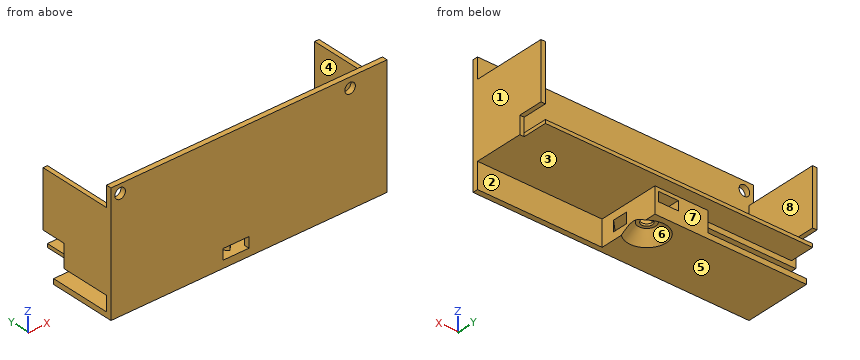
Autodesk Inventor part; units mm, degrees
ref_plane "Work Plane1" through (-11.25, -9.75, 3.625) normal (0, 0, -1) x (-1, 0, 0)
ref_plane "YZ Plane" through (0, 0, 0) normal (1, 0, 0) x (0, 1, 0)
ref_plane "XZ Plane" through (0, 0, 0) normal (0, 1, 0) x (-1, 0, 0)
sketch "Sketch1" plane through (0, 0, 0) normal (0, 0, 1) x (1, 0, 0)
  line L0 (-39.25, 11.25) -> (39.25, 11.25)
  line L1 (39.25, 11.25) -> (39.25, -11.25)
  line L2 (39.25, -11.25) -> (-39.25, -11.25)
  line L3 (-39.25, -11.25) -> (-39.25, 11.25)
  line L4 (-39.25, -11.25) -> (39.25, -11.25)
  line L5 (39.25, -11.25) -> (39.25, -9.75)
  line L6 (39.25, -9.75) -> (-39.25, -9.75)
  line L7 (-39.25, -9.75) -> (-39.25, -11.25)
  point P0 (0, 0)
  point P1 (0, 11.25)
  point P2 (39.25, 0)
  point P3 (-39.25, -9.75)
  dimension "d0" = 22.5
  dimension "d1" = 78.5
  dimension "d2" = 1.5
extrude "Extrusion1" add sketch "Sketch1" along normal blind 33 contours L6 L1 L2 L3
sketch "Sketch2" plane through (-39.25, -9.75, 0) normal (0, 1, 0) x (1, 0, 0)
  line L0 (0, -1.5) -> (28, -1.5)
  line L1 (28, -1.5) -> (28, -5.75)
  line L2 (28, -5.75) -> (0, -5.75)
  line L3 (0, -5.75) -> (0, -1.5)
  line L4 (0, 0) -> (0, -33)
  line L5 (78.5, 0) -> (0, 0)
  line L6 (0, -5.75) -> (29.5, -5.75)
  line L7 (29.5, -5.75) -> (29.5, -7.25)
  line L8 (29.5, -7.25) -> (0, -7.25)
  line L9 (0, -7.25) -> (0, -5.75)
  line L10 (0, 0) -> (78.5, 0)
  line L11 (29.5, -7.25) -> (28, -7.25)
  line L12 (28, -7.25) -> (28, 0)
  line L13 (28, 0) -> (29.5, 0)
  line L14 (29.5, 0) -> (29.5, -7.25)
  line L15 (0, -33) -> (78.5, -33)
  line L16 (1.25, -33) -> (77.25, -33)
  line L17 (77.25, -28.25) -> (77.25, -8.25)
  line L18 (77.25, -8.25) -> (1.25, -8.25)
  line L19 (1.25, -8.25) -> (1.25, -28.25)
  line L20 (0, 0) -> (0, -33)
  line L21 (0, -7.25) -> (78.5, -7.25)
  line L22 (78.5, 0) -> (78.5, -33)
  line L23 (43.075, -2.6) -> (35.425, -2.6)
  line L24 (35.425, -2.6) -> (35.425, -7.25)
  line L25 (35.425, -7.25) -> (43.075, -7.25)
  line L26 (43.075, -7.25) -> (43.075, -2.6)
  line L27 (42.075, -3.6) -> (36.425, -3.6)
  line L28 (36.425, -3.6) -> (36.425, -6.25)
  line L29 (36.425, -6.25) -> (42.075, -6.25)
  line L30 (42.075, -6.25) -> (42.075, -3.6)
  line L31 (29.5, -7.25) -> (35.425, -7.25)
  line L32 (43.075, -2.6) -> (43.075, 0)
  line L33 (77.25, -28.25) -> (1.25, -28.25)
  line L34 (77.25, -28.25) -> (78.5, -28.25)
  line L35 (1.25, -28.25) -> (0, -28.25)
  line L36 (0, -33) -> (78.5, -33)
  line L37 (78.5, -33) -> (78.5, -34)
  line L38 (78.5, -34) -> (0, -34)
  line L39 (0, -34) -> (0, -33)
  point P0 (39.25, 0)
  point P1 (39.25, -8.25)
  point P2 (39.25, 0)
  point P3 (39.25, -7.25)
  point P4 (39.25, -6.25)
  point P5 (42.075, -4.925)
  point P6 (43.075, -4.925)
  point P7 (0, -1.5)
  point P8 (0, -5.75)
  point P9 (0, -7.25)
  point P10 (0, -7.25)
  dimension "d5" = 28
  dimension "d6" = 4.25
  dimension "d7" = 1.5
  dimension "d8" = 1.5
  dimension "d9" = 1.5
  dimension "d10" = 20
  dimension "d11" = 76
  dimension "d12" = 1
  dimension "d13" = 4.65
  dimension "d14" = 7.65
  dimension "d16" = 2.65
  dimension "d17" = 5.65
  dimension "d52" = 1
extrude "Extrusion2" add sketch "Sketch2" along normal blind 17.5 contours L4 L5 L12 L0 | L12 L5 L14 L6 L1 | L2 L12 L8 L4 | L6 L7 L8 L12
extrude "Extrusion3" add sketch "Sketch2" along normal blind 21 contours L8 L21 L22 L34 L17 L18 L19 L35 L4
extrude "Extrusion4" add sketch "Sketch2" along normal blind 17.5 contours L14 L5 L32 L23 L24 L21 L7 | L24 L23 L26 L21
sketch "Sketch3" plane through (-38, -9.75, 8.25) normal (0, 0, 1) x (1, 0, 0)
  line L0 (75.85, 20.7) -> (0.15, 20.7)
  line L1 (0.15, 20.7) -> (0.15, 0)
  line L2 (0.15, 0) -> (75.85, 0)
  line L3 (75.85, 0) -> (75.85, 20.7)
  line L4 (76, 0) -> (0, 0)
  circle A0 centre (38, 10.35) radius 1.575
  line L5 (76, 0) -> (0, 0)
  point P0 (38, 9.75)
  point P1 (38, 20.7)
  point P2 (75.85, 10.35)
  dimension "d24" = 75.7
  dimension "d25" = 20.7
  dimension "d28" = 3.15
extrude "Extrusion5" [suppressed]
sketch "Sketch4" plane through (2.825, -9.75, 6.25) normal (0, 0, -1) x (-1, 0, 0)
  line L0 (5.65, 0) -> (0, 0)
  line L1 (5.65, 0) -> (5.65, 17.5)
  line L2 (0, 17.5) -> (5.65, 17.5)
  line L3 (0, 0) -> (0, 17.5)
  line L4 (2.825, 7.1746) -> (0, 8.8056)
  line L5 (0.075, 8.7623) -> (0.075, 11.9377)
  line L6 (0.075, 11.9377) -> (2.825, 13.5254)
  line L7 (2.825, 13.5254) -> (5.575, 11.9377)
  line L8 (5.575, 11.9377) -> (5.575, 8.7623)
  line L9 (5.65, 8.8056) -> (2.825, 7.1746)
  circle A0 centre (2.825, 10.35) radius 1.575
  point P0 (2.825, 9.75)
  point P1 (5.575, 10.35)
  point P2 (2.825, 0)
  dimension "d31" = 5.5
  dimension "d34" = 3.15
  dimension "d37" = 10.35
extrude "Extrusion6" add sketch "Sketch4" along normal up to surface (2.65 mm away) contours L0 L3 L4 L9 L1
extrude "Extrusion7" cut sketch "Sketch4" along normal mid plane 10 contours A0
fillet "Fillet1" [suppressed]
sketch "Sketch6" plane through (0, 0, 0) normal (0, 0, -1) x (-1, 0, 0)
  circle A0 centre (0, 0.6) radius 2.5
  line L0 (39.25, -11.25) -> (-39.25, -11.25)
  line L1 (39.25, 7.75) -> (39.25, -11.25)
  point P0 (0, 0)
  dimension "d43" = 5
  dimension "d44" = 11.85
  dimension "d45" = 39.25
extrude "Extrusion8" cut sketch "Sketch6" against normal blind 3
chamfer "Chamfer1" distance 3 angle 45 1 edges at (2.5, 0.6, 0)
extrude "Extrusion9" add sketch "Sketch2" against normal up to surface (1.5 mm away) contours L15 L37 L38 L39
sketch "Sketch7" plane through (-11.25, -9.75, 1.5) normal (-1, 0, 0) x (0, 0, 1)
  line L0 (0.625, 9) -> (3.625, 9)
  line L1 (3.625, 9) -> (3.625, 4)
  line L2 (3.625, 4) -> (0.625, 4)
  line L3 (0.625, 4) -> (0.625, 9)
  line L4 (4.25, 0) -> (0, 0)
  line L5 (0, 0) -> (4.25, 0)
  point P0 (-1.5, 9.75)
  point P1 (2.125, 4)
  point P2 (2.125, 0)
  dimension "d55" = 4
  dimension "d56" = 3
  dimension "d57" = 5
sketch "Sketch8" plane through (-39.25, -11.25, 0) normal (0, -1, 0) x (1, 0, 0)
  line L0 (41.75, 2) -> (36.75, 2)
  line L1 (36.75, 2) -> (36.75, 5)
  line L2 (36.75, 5) -> (41.75, 5)
  line L3 (41.75, 5) -> (41.75, 2)
  line L4 (0, 0) -> (78.5, 0)
  point P0 (39.25, 0)
  point P1 (39.25, 2)
  point P2 (39.25, 0)
  dimension "d58" = 5
  dimension "d59" = 3
  dimension "d60" = 2
loft "Loft1" [suppressed]
sketch "Sketch9" plane through (39.25, 11.25, 7.25) normal (0, 0, -1) x (-1, 0, 0)
  line L0 (0, -21) -> (0, 0)
  line L1 (0, 0) -> (1.25, 0)
  line L2 (1.25, 0) -> (1.25, -7)
  line L3 (1.25, -7) -> (0, -7)
  line L4 (0, -7) -> (0, 0)
  line L5 (0, 0) -> (78.5, 0)
  point P0 (39.25, -11.25)
  point P1 (0, -7)
  dimension "d65" = 7
extrude "Extrusion10" cut sketch "Sketch9" against normal blind 5
mirror "Mirror1" about plane through (0, 0, 0) normal (1, 0, 0) of "Extrusion10"
sketch "Sketch10" plane through (-39.25, -11.25, 0) normal (-1, 0, 0) x (0, 0, 1)
  line L0 (12.25, 15.5) -> (7.25, 15.5)
  line L1 (1.5, 19) -> (5.75, 19)
  line L2 (5.75, 19) -> (7.25, 19)
  line L3 (7.25, 19) -> (7.25, 15.5)
  line L4 (7.25, 15.5) -> (5.75, 15.5)
  line L5 (5.75, 15.5) -> (5.75, 19)
  point P0 (0, 11.25)
extrude "Extrusion11" cut sketch "Sketch10" against normal up to surface (28 mm away)
ref_plane "Work Plane1" through (-11.25, -9.75, 3.625) normal (0, 0, -1) x (-1, 0, 0)
sketch "Sketch11" plane through (-11.25, -9.75, 3.625) normal (0, 0, -1) x (-1, 0, 0)
  line L0 (0, 0) -> (0, 14)
  line L1 (0, 17.5) -> (0, 14)
  line L2 (0, 0) -> (0, 17.5)
  line L3 (-15.075, 0) -> (-15.075, 6.3979)
  line L4 (-15.075, 6.3979) -> (-9.6656, 6.3979) construction
  line L5 (-7.5375, 0.5) -> (-16.6978, 9.6603)
  line L6 (-7.5375, 0.5) -> (5.4171, 0.5) construction
  line L7 (-15.075, 17.5) -> (0, 17.5)
  line L8 (-7.5375, 0.5) -> (0, 8.0375)
  line L9 (0, 0) -> (0, 14)
  line L10 (-7.5375, 0.5) -> (3.1221, 0.5) construction
  line L11 (-18.8191, 7.5389) -> (-7.5375, -3.7426)
  line L12 (-7.5375, -3.7426) -> (2.1213, 5.9162)
  line L13 (-49.25, 0) -> (26.75, 0)
  line L14 (0, 3.7949) -> (0, 8.0375)
  line L15 (-15.075, 3.7949) -> (-15.075, 8.0375)
  line L16 (-11.25, 0) -> (-11.25, -1.5)
  line L17 (-3.7949, 0) -> (-3.7949, -1.5)
  line L18 (-11.25, -1.5) -> (-3.7949, -1.5)
  line L19 (-11.25, -1.5) -> (-3.7949, -1.5)
  line L20 (-3.7949, -1.5) -> (-3.7949, -2.3604)
  line L21 (-3.7949, -2.3604) -> (-11.25, -2.3604)
  line L22 (-11.25, -2.3604) -> (-11.25, -1.5)
  line L23 (28, -1.5) -> (-50.5, -1.5)
  point P0 (-11.25, 9.75)
  point P1 (-7.5375, 17.5)
  point P2 (0, 3.7949)
  point P3 (0, 8.0375)
  point P4 (-11.2801, 0)
  dimension "d73" = 135
  dimension "d74" = 45
  dimension "d75" = 3
  dimension "d76" = 0.5
extrude "Extrusion12" cut sketch "Sketch11" along normal mid plane 3 contours L12 L13 L11 L3 L15 L5 L8 L0 | L17 L18 L12 | L12 L18 L11 L16 L13 | L18 L20 L21 L12 | L12 L21 L11 L18 | L18 L16 L11 | L11 L21 L22 L18
sketch "Sketch12" plane through (-38, -9.75, 8.25) normal (0, 1, 0) x (1, 0, 0)
  circle A0 centre (1.37, -23.25) radius 1.5
  line L0 (-1.25, -25.75) -> (77.25, -25.75)
  line L1 (-1.25, -20) -> (-1.25, -25.75)
  circle A1 centre (66.75, -22.875) radius 1.5
  line L2 (77.25, -20) -> (77.25, -25.75)
  point P0 (38, 8.25)
  dimension "d79" = 3
  dimension "d80" = 2.5
  dimension "d81" = 2.62
  dimension "d82" = 3
  dimension "d83" = 2.875
  dimension "d84" = 10.5
extrude "Extrusion13" cut sketch "Sketch12" against normal up to surface (1.5 mm away)
sketch "Sketch13" plane through (-38, -9.75, 8.25) normal (0, 1, 0) x (1, 0, 0)
  circle A0 centre (1.37, -23.25) radius 1.5
  circle A1 centre (66.75, -22.875) radius 1.5
  line L0 (77.25, -20) -> (76, -20)
  line L1 (76, -20) -> (76, 0)
  line L2 (76, 0) -> (0, 0)
  line L3 (0, 0) -> (0, -20)
  line L4 (0, -20) -> (-1.25, -20)
  line L5 (-1.25, -20) -> (-1.25, -25.75)
  line L6 (-1.25, -25.75) -> (77.25, -25.75)
  line L7 (77.25, -20) -> (77.25, -25.75)
  point P0 (38, 8.25)
Could you check a few things on this model? Use its own coordinates, in mm. Face numbers are marked on the shaded views. A direction names the side the tool comes from. Coordinates: 2 decimals unless noted, no trailing zeros. Write each loop counter-clockwise with the first axis right and the second up, starting at its lowest first coordinate (ties: lowest second). Pieces come first, ordered by that corner, then holes. Notation, with made-up numbers: (80, 30) -> (106, 30) arc R32 cw to (106, 57) -> close; hole circle Ø2 at (44, 15.5). An arc over 180 degrees is marked (long way). Return JSON: item names as keys, results as strings.
(1) I'm going to push flat-ended pins straight in: pin 1 (1.3 mm diameter, centred on x = -21, z = 3, fed in from +Y); pin 2 (6.5 mm diameter, centred on x = -4, y = -4.5, fed in from -Z); pin 3 (1 mm diameter, centred on y = 3.5, z = 5.5, fed in from +X) (3 decimals); pin 4 (4 mm diameter, centred on x = 0, y = 0.6, fed in from +Z). Where does each tip first touch, or does it pass through?
Numbers:
{"pin 1": "stops at y = -9.75", "pin 2": "stops at z = 0", "pin 3": "stops at x = 3.825", "pin 4": "stops at z = 8.25"}
(2) I need wall thicknesses on L1, parallel to Z at x = -23.5, y = -9.25; L2, parallel to X at y = -5.75, z = 14; L3, parallel to Z at x = 28.75, y = -10.75 (3 decimals). Which ranges of each line are inside material? Lowest first, please.
Numbers:
{"L1": "z = 0 to 1.5, 5.75 to 8.25", "L2": "x = -39.25 to -38, 38 to 39.25", "L3": "z = 0 to 29.625, 32.625 to 34"}
(3) Which directions (+Z, -Z, +X, -X, +Y, -Y) give clear straight access to the entire face, cutting with the end or side of a thin tool? Please do the marked faces 1, 2, 3, 4 and 5.
Numbers:
{"face 1": "+Z, -Z, +X, +Y, -Y", "face 2": "-Z, +X, +Y", "face 3": "+Y", "face 4": "+Z, +Y", "face 5": "-Z, +X, -X, +Y, -Y"}
(4) Imagine slicing it at A-A, the plane x = 28.75. Please give me the cut outline in (y, z) (3 decimals).
Numbers:
{"outline": "(-11.25, 0) -> (-9.75, 0) -> (-9.75, 7.25) -> (11.25, 7.25) -> (11.25, 8.25) -> (-9.75, 8.25) -> (-9.75, 29.625) -> (-11.25, 29.625) -> close; (-11.25, 32.625) -> (-9.75, 32.625) -> (-9.75, 34) -> (-11.25, 34) -> close"}
(5) Imagine slicing it at B-B, the plane z = 20.5. Please give me the cut outline in (x, y).
Numbers:
{"outline": "(-39.25, -11.25) -> (39.25, -11.25) -> (39.25, 11.25) -> (38, 11.25) -> (38, -9.75) -> (-38, -9.75) -> (-38, 11.25) -> (-39.25, 11.25) -> close"}
(6) We'd pull the mould along Y, two halves only. Please class the marked faces 6, 7 and 8: +Y half, -Y half, draft (parallel to the pull), parting line (faces both ways), or undercut.
Numbers:
{"face 6": "undercut", "face 7": "+Y half", "face 8": "draft"}
(7) Imagine slicing it at C-C, the plane x = -20. Please give me the cut outline in (y, z), then the cut area to 3 significant figures.
Numbers:
{"outline": "(-11.25, 0) -> (7.75, 0) -> (7.75, 1.5) -> (-9.75, 1.5) -> (-9.75, 5.75) -> (4.25, 5.75) -> (4.25, 7.25) -> (11.25, 7.25) -> (11.25, 8.25) -> (-9.75, 8.25) -> (-9.75, 34) -> (-11.25, 34) -> close", "area": "119 mm2"}
